Autodesk Inventor part; units mm, degrees
ref_plane "YZ Plane" through (0, 0, 0) normal (1, 0, 0) x (0, 1, 0)
ref_plane "XZ Plane" through (0, 0, 0) normal (0, 1, 0) x (-1, 0, 0)
ref_plane "XY Plane" through (0, 0, 0) normal (0, 0, 1) x (1, 0, 0)
sketch "Sketch1" plane through (0, 0, 0) normal (0, 1, 0) x (-1, 0, 0)
  circle A0 centre (0, 0) radius 12.5
  line L0 (25, -40) -> (-25, -40)
  line L1 (-25, -40) -> (-25, 27)
  line L2 (-25, 27) -> (25, 27)
  line L3 (25, 27) -> (25, -40)
  point P0 (0, -40)
  dimension "d0" = 25
  dimension "d1" = 50
  dimension "d2" = 67
  dimension "d3" = 40
extrude "Extrusion1" add sketch "Sketch1" along normal mid plane 2
fillet "Fillet1" radius 12 2 edges at (25, 0, 27) (-25, 0, 27)
properties part number "bracket"
Design review of the part built by this model. Coordinates are the model's own, in mm. Give positions to 0.01 mm unless a question says otherwise; leave off trailing zeros. Write each loop counter-clockwise with the first axis right and the second up, starting at its lowest first coordinate (ties: lowest second). Pieces come first, ordered by that corner, then holes. Notation, with made-up numbers: (7.5, -10) - (42.5, -10) arc R6 ccw to (42.5, -1) - close; hole circle Ø5 at (64, 39.25). An arc over 180 degrees is marked (long way). Return JSON: item names as keys, results as strings. Group by question number.
(1) We need section C-C, the plane y = -0.7. Give the boundary of the cut face in (x, z).
(2) To check wall thickness, follow probe 1 along Z at (x, y) = (0, 0); probe 2 along Z at (x, y) = (-13.5, 0.35); probe 3 along Z at (x, y) = (-18, 0.9). State the ranges of each line that lie inside material, in increasing order.
(3) We need section D-D, the plane z = 19. Give the boundary of the cut face in (x, y), then the cut area to 3 significant figures.
(4) We need section B-B, the plane z = 0. Give the boundary of the cut face in (x, y).
(5) We need section A-A, the plane x = 0. Give the boundary of the cut face in (y, z), then the cut area to 3 significant figures.
Reported:
{
 "1": {"outline": "(-25, -40) - (25, -40) - (25, 15) arc R12 ccw to (13, 27) - (-13, 27) arc R12 ccw to (-25, 15) - close; hole circle Ø25 at (0, 0)"},
 "2": {"probe 1": "z = -40 to -12.5, 12.5 to 27", "probe 2": "z = -40 to 26.99", "probe 3": "z = -40 to 25.91"},
 "3": {"outline": "(-24.31, -1) - (24.31, -1) - (24.31, 1) - (-24.31, 1) - close", "area": "97.3 mm2"},
 "4": {"outline": "(-25, -1) - (-12.5, -1) - (-12.5, 1) - (-25, 1) - close; (12.5, -1) - (25, -1) - (25, 1) - (12.5, 1) - close"},
 "5": {"outline": "(-1, -40) - (1, -40) - (1, -12.5) - (-1, -12.5) - close; (-1, 12.5) - (1, 12.5) - (1, 27) - (-1, 27) - close", "area": "84.0 mm2"}
}
